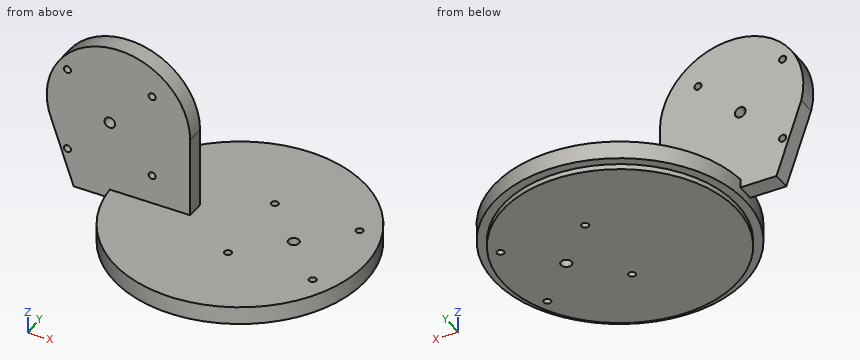
Autodesk Fusion 360 part; units mm, degrees
sketch "Sketch1" plane through (0, 0, 0) normal (0, 0, 1) x (1, 0, 0)
  circle A0 centre (0, 0) radius 70
  dimension "d1" = 140
extrude "Extrude1" add sketch "Sketch1" along normal blind 10
sketch "Sketch2" plane through (0, 0, 0) normal (0, 0, -1) x (1, 0, 0)
  circle A0 centre (0, 0) radius 70
  circle A1 centre (0, 0) radius 65
  dimension "d4" = -5
extrude "Extrude2" add sketch "Sketch2" along normal blind 3 contours A1
sketch "Sketch3" plane through (0, 0, 0) normal (0, 1, 0) x (1, 0, 0)
  line L0 (-25, -55) -> (-25, -5)
  line L1 (-25, -5) -> (-90, -5)
  line L2 (-90, -5) -> (-103.8281, -45.3888)
  arc A0 (-103.8281, -45.3888) -> (-25, -55) centre (-65, -55) ccw
  dimension "d7" = 50
  dimension "d8" = 65
  dimension "d9" = 40
  dimension "d12" = 5
  dimension "d14" = 25
extrude "Extrude3" add sketch "Sketch3" along normal mid plane 10
sketch "Sketch4" plane through (0, 0, 10) normal (0, 0, 1) x (-1, 0, 0)
  line L0 (69.8212, -5) -> (25, -5)
  line L1 (25, -5) -> (25, 5)
  line L2 (25, 5) -> (69.8212, 5)
  arc A0 (69.8212, 5) -> (69.8212, -5) centre (0, 0) ccw
  line L3 (-6.378, 23.622) -> (-53.622, 23.622)
  line L4 (-53.622, 23.622) -> (-53.622, -23.622)
  line L5 (-53.622, -23.622) -> (-6.378, -23.622)
  line L6 (-6.378, -23.622) -> (-6.378, 23.622)
  line L7 (-6.378, 23.622) -> (-53.622, -23.622) construction
  line L8 (-53.622, 23.622) -> (-6.378, -23.622) construction
  point P0 (-30, 0)
  dimension "d17" = 47.244
  dimension "d18" = 47.244
  dimension "d20" = 30
hole "Hole1" at (6.378, 23.622, 10) at (53.622, 23.622, 10) at (53.622, -23.622, 10) at (6.378, -23.622, 10) direction (0, 0, -1) diameter 4 depth 15 tip angle 118
hole "Hole2" at (30, 0, 10) direction (0, 0, -1) diameter 6 depth 15 tip angle 118
sketch "Sketch5" plane through (0, -5, 0) normal (0, -1, 0) x (1, 0, 0)
  line L0 (-69.8212, 10) -> (-25, 10)
  line L1 (-25, 10) -> (-25, 55)
  arc A0 (-25, 55) -> (-103.8281, 45.3888) centre (-65, 55) ccw
  line L2 (-103.8281, 45.3888) -> (-90, 5)
  line L3 (-90, 5) -> (-69.8212, 5)
  line L4 (-69.8212, 5) -> (-69.8212, 10)
  line L5 (-93.4432, 73.622) -> (-46.1992, 73.622)
  line L6 (-46.1992, 73.622) -> (-46.1992, 26.378)
  line L7 (-46.1992, 26.378) -> (-93.4432, 26.378)
  line L8 (-93.4432, 26.378) -> (-93.4432, 73.622)
  line L9 (-93.4432, 73.622) -> (-46.1992, 26.378) construction
  line L10 (-46.1992, 73.622) -> (-93.4432, 26.378) construction
  point P0 (-69.8212, 50)
  dimension "d27" = 47.244
  dimension "d28" = 47.244
  dimension "d30" = 45
hole "Hole3" at (-93.4432, -5, 73.622) at (-46.1992, -5, 73.622) at (-93.4432, -5, 26.378) at (-46.1992, -5, 26.378) direction (0, 1, 0) diameter 4 depth 15 tip angle 118
hole "Hole4" at (-69.8212, -5, 50) direction (0, 1, 0) diameter 6 depth 15 tip angle 118
Check sheet for the modelled part. Datum: model origin and axes. Units: mm. Coordinates: 2 decimals unless noted, no trailing zeros. Loops run counter-clockwise (first coordinate to the right, second up) from the corner with the lowest first, then second, coordinate; pieces in that order, holes last.
1) Gauge pin test, flat ends, axial feed: pin 1 (4 mm diameter, centred on x = -8.5, y = -32, fed in from +Z); pin 2 (4.5 mm diameter, centred on x = -46.2, z = 73.62, fed in from -Y); pin 3 (5 mm diameter, centred on x = -75, y = 0, fed in from -Z). Record the tip position at first contact, or that the pin passes through.
2) Material ranges on probe 1 along Z at (x, y) = (3, 63.5); probe 2 along Y at (x, z) = (-58, 14); probe 3 along Z at (x, y) = (31, -58), recorded low to high.
3) Sectioned sample at C-C (z = 50). Record the boundary of the cut face in (x, y).
4) Sectioned sample at B-B (x = 0). Record the boundary of the cut face in (y, z), and give its area (3 significant figures).
5) Sectioned sample at A-A (y = 0). Record the boundary of the cut face in (x, z), and give its area (3 significant figures).
6) Sectioned sample at D-D (x = 30). Record the boundary of the cut face in (y, z), and give its area (3 significant figures).
Check sheet entries:
1. pin 1: stops at z = 10
1. pin 2: stops at y = -5
1. pin 3: stops at z = 5
2. probe 1: z = -3 to 10
2. probe 2: y = -5 to 5
2. probe 3: z = 0 to 10
3. outline: (-104.69, -5) - (-72.82, -5) - (-72.82, 5) - (-104.69, 5) - close; (-66.82, -5) - (-25, -5) - (-25, 5) - (-66.82, 5) - close
4. outline: (-70, 0) - (-65, 0) - (-65, -3) - (65, -3) - (65, 0) - (70, 0) - (70, 10) - (-70, 10) - close
4. area: 1,790 mm2
5. outline: (-103.83, 45.39) - (-90, 5) - (-70, 5) - (-70, 0) - (-65, 0) - (-65, -3) - (27, -3) - (27, 10) - (-25, 10) - (-25, 55) arc R40 ccw (long way) to start; (33, -3) - (65, -3) - (65, 0) - (70, 0) - (70, 10) - (33, 10) - close; hole circle Ø4 at (-93.44, 26.38); hole circle Ø4 at (-93.44, 73.62); hole circle Ø6 at (-69.82, 50); hole circle Ø4 at (-46.2, 26.38); hole circle Ø4 at (-46.2, 73.62)
5. area: 7,590 mm2
6. outline: (-63.25, 0) - (-57.66, 0) - (-57.66, -3) - (-3, -3) - (-3, 10) - (-63.25, 10) - close; (3, -3) - (57.66, -3) - (57.66, 0) - (63.25, 0) - (63.25, 10) - (3, 10) - close
6. area: 1,530 mm2
